Here's how the part is built. I have some questions about the finished solid (model axes, mm). Face numbers are marked on the shaded views. Round coordinates to 2 decimals unless told otherwise and drop trailing zeros. Write each loop counter-clockwise with the first axis right and the second up, starting at its lowest first coordinate (ties: lowest second). Pieces come first, ordered by that corner, then holes. Notation, with made-up numbers: (89, 0) - (133, 0) arc R17 ccw to (133, 9) - close; hole circle Ø5 at (76, -2). An arc over 180 degrees is marked (long way). Return JSON: item names as keys, results as strings. Group by question number.
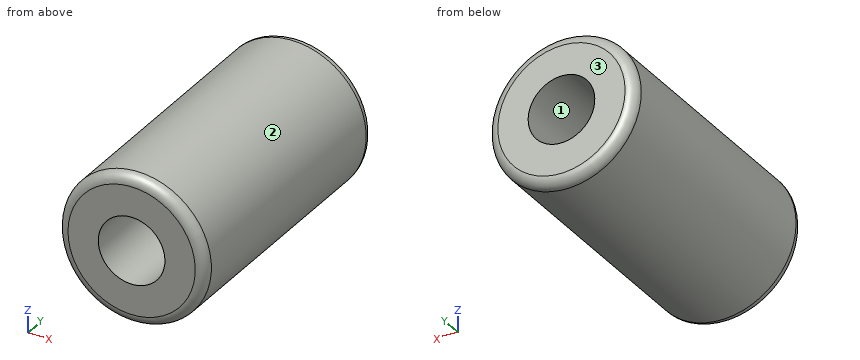
Autodesk Inventor part; units mm, degrees
ref_plane "YZ Plane" through (0, 0, 0) normal (1, 0, 0) x (0, 1, 0)
ref_plane "XZ Plane" through (0, 0, 0) normal (0, 1, 0) x (-1, 0, 0)
ref_plane "XY Plane" through (0, 0, 0) normal (0, 0, 1) x (1, 0, 0)
sketch "スケッチ1" plane through (0, 0, 0) normal (0, 1, 0) x (-1, 0, 0)
  circle A0 centre (0, 0) radius 3.65
  dimension "d0" = 7.3
extrude "押し出し1" add sketch "スケッチ1" along normal blind 13.8
sketch "スケッチ2" plane through (0, 13.8, 0) normal (0, 1, 0) x (1, 0, 0)
  point P0 (0, 0)
  point P1 (0, 0)
hole "穴1" at (0, 13.8, 0) direction (0, -1, 0) diameter 3.3 end through all
fillet "フィレット1" radius 0.5 2 edges at (3.65, 0, 0) (3.65, 13.8, 0)
properties part number "spacer_for_frame"
1) Imagine slicing it at A-A (z = 0). Please give me the cut outline in (x, y), plus the area to 3 significant figures.
2) Imagine slicing it at C-C (y = 7). Please give me the cut outline in (x, z), plus the area to 3 significant figures.
3) Will these pins go through, and if not, where does the flat tip stop? pin 1 Ø1 at (y, z) = (10.5, -3) entering from -X; pin 2 Ø2 at (y, z) = (9.5, 2) entering from -X.
4) I need wall thicknesses on line 1 along Z through (x, y) = (0, 5.75); line 2 along Z through (x, y) = (1.5, 2); line 3 along X through (y, z) = (5.5, 0.5). Which ranges of each line are inside material? Lowest first, please.
5) If we mould it in two halves opening along X, with no side actions, what happens to the marked faces 1, 2 and 3? For each: released by +X, released by -X, zero draft, split by the parting line, or undercut.
6) Imagine slicing it at B-B (x = 0). Please give me the cut outline in (y, z).
Results found:
{
 "1": {"outline": "(-3.65, 0.5) arc R0.5 ccw to (-3.15, 0) - (-1.65, 0) - (-1.65, 13.8) - (-3.15, 13.8) arc R0.5 ccw to (-3.65, 13.3) - close; (1.65, 0) - (3.15, 0) arc R0.5 ccw to (3.65, 0.5) - (3.65, 13.3) arc R0.5 ccw to (3.15, 13.8) - (1.65, 13.8) - close", "area": "55.0 mm²"},
 "2": {"outline": "circle Ø7.3 at (0, 0); hole circle Ø3.3 at (0, 0)", "area": "33.3 mm²"},
 "3": {"pin 1": "stops at x = -2.66", "pin 2": "stops at x = -3.51"},
 "4": {"line 1": "z = -3.65 to -1.65, 1.65 to 3.65", "line 2": "z = -3.33 to -0.69, 0.69 to 3.33", "line 3": "x = -3.62 to -1.57, 1.57 to 3.62"},
 "5": {"face 1": "undercut", "face 2": "split by the parting line", "face 3": "zero draft"},
 "6": {"outline": "(0, -3.15) arc R0.5 ccw to (0.5, -3.65) - (13.3, -3.65) arc R0.5 ccw to (13.8, -3.15) - (13.8, -1.65) - (0, -1.65) - close; (0, 1.65) - (13.8, 1.65) - (13.8, 3.15) arc R0.5 ccw to (13.3, 3.65) - (0.5, 3.65) arc R0.5 ccw to (0, 3.15) - close"}
}
